The figure shows three views and two pictorial views of one solid part (mm, origin at its lowest corner). Answer the questions. A direction names the side the tool comes from. Coordinates: 2 decimals unless noted, no trailing zeros. Order: outer loops, then holes, each group sorted by start corner. A loop starts at its lowest first (then second) coordinate and runs counter-clockwise, first axis right, second up. Notation, with made-up numbers: M 62.5,45 L 90.5,45 A20 ccw 90.5,77 Z; hole C -9,3 d11. An arc over 180 degrees is marked long. Answer in a Markdown table with one row per item. Add a question column.
Item 1: Which of the six approach directions +Z, -Z, +X, -X, +Y, -Y give full straight-line access (tool end or side, diameter ignored) to the marked faces 1, 2 and 3?
Item 2: The part is cut by section A-A (y = 41). Write down the section's boundary in (x, z).
Item 3: The part is cut by section B-B (z = 5). Write down the section's boundary in (x, y).
Item 4: The part is cut by section D-D (x = 4.75). Write down the section's boundary in (y, z).
Item 5: The part is cut by section C-C (z = 7). Write down the section's boundary in (x, y).
Item 6: Flat-ended cylindrical pins translate along their axes: pin 1 Ø1 at (x, z) = (16.5, 3.5) entering from +Y; pin 2 Ø5 at (x, z) = (2.5, 3) entering from -Y; pin 3 Ø1.5 at (x, y) = (3.5, 21) entering from -Z (3 decimals); pin 4 Ø2 at (x, z) = (18, 5) entering from -Y. Find the tip coordinate at first contact, or state that the pin passes through.
Item 7: Consider line 1 (Z direction, x = 1.5, y = 41); line 2 (Y direction, x = 6.5, z = 4.5); line 3 (Y direction, x = 20.5, z = 6.5). Determine where each line is inside the solid, lowest interval first. Write a range as from..to.
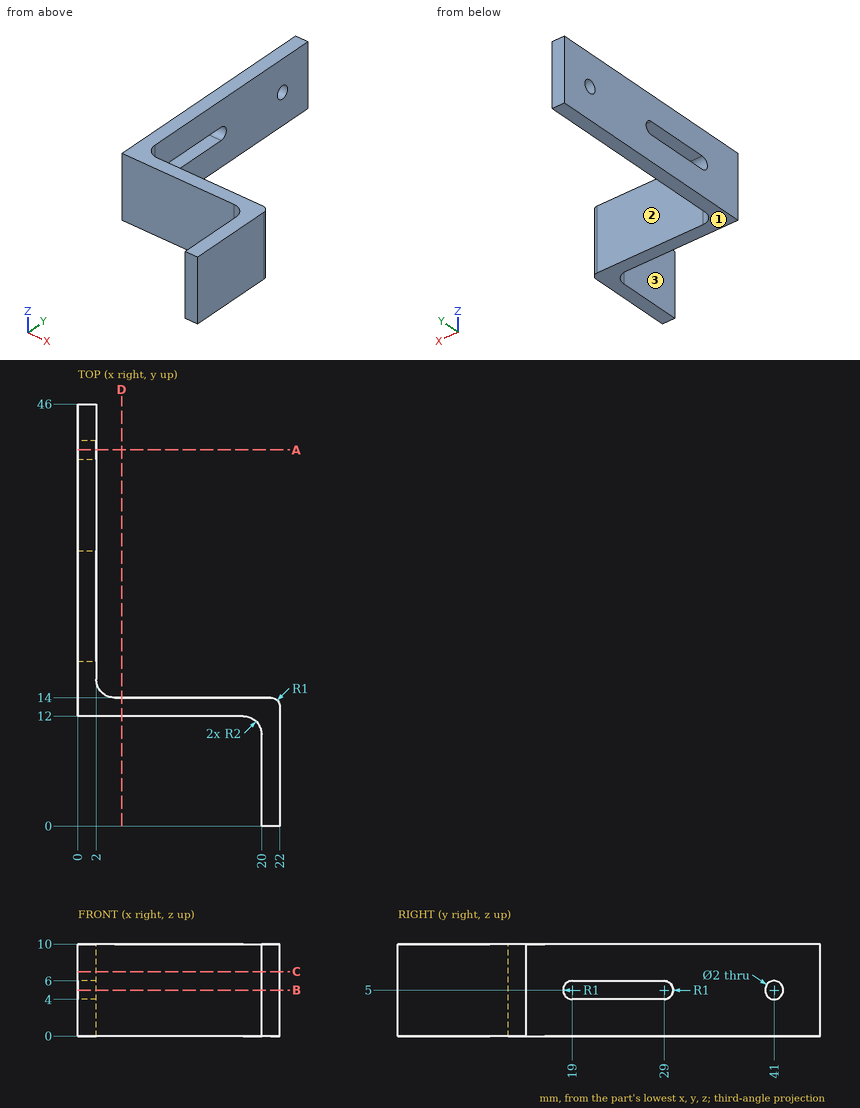
Reply:
| question | item | result |
|---|---|---|
| 1 | face 1 | -Z, +X, -X, +Y, -Y |
| 1 | face 2 | +Z, -Z, +X, +Y |
| 1 | face 3 | +Z, -Z, -X, -Y |
| 2 | outline | M 0,0 L 2,0 L 2,4 L 0,4 Z; M 0,6 L 2,6 L 2,10 L 0,10 Z |
| 3 | outline | M 0,12 L 18,12 A2 cw 20,10 L 20,0 L 22,0 L 22,13 A1 ccw 21,14 L 4,14 A2 cw 2,16 L 2,18 L 0,18 Z; M 0,30 L 2,30 L 2,40 L 0,40 Z; M 0,42 L 2,42 L 2,46 L 0,46 Z |
| 4 | outline | M 12,0 L 14,0 L 14,10 L 12,10 Z |
| 5 | outline | M 0,12 L 18,12 A2 cw 20,10 L 20,0 L 22,0 L 22,13 A1 ccw 21,14 L 4,14 A2 cw 2,16 L 2,46 L 0,46 Z |
| 6 | pin 1 | stops at y = 14 |
| 6 | pin 2 | stops at y = 12 |
| 6 | pin 3 | passes through |
| 6 | pin 4 | stops at y = 11.73 |
| 7 | line 1 | z = 0..4, 6..10 |
| 7 | line 2 | y = 12..14 |
| 7 | line 3 | y = 0..14 |
